The model under review builds one solid part; all positions refer to its coordinate system, in mm. A direction names the side the tool comes from. Round coordinates to 2 decimals unless told otherwise and drop trailing zeros. Write each loop counter-clockwise with the first axis right and the second up, starting at its lowest first coordinate (ties: lowest second). Pieces come first, ordered by that corner, then holes. Notation, with made-up numbers: (6, 74.5) - (30, 74.5) arc R20 cw to (30, 86.5) - close; hole circle Ø6 at (-32.75, 14.25). An arc over 180 degrees is marked (long way). Use one line per item in the form item = value.
from build123d import *

# Parameters (mm, degrees)
SKETCH1_W           = 20
SKETCH1_H           = 4.5
SKETCH2_R           = 1.5
CUT_EXTRUDE1_DEPTH  = 3
CHAMFER1_SIZE       = 0.3
SKETCH3_R           = 0.5
BOSS_EXTRUDE1_DEPTH = 5


with BuildPart() as part:
    # Sketch1 → Revolve1 (revolve)
    with BuildSketch(Plane(origin=(0, 0, 0), x_dir=(0, 0, -1), z_dir=(1, 0, 0)), mode=Mode.PRIVATE) as revolve1_sk:
        with Locations((0, 2.25)):
            Rectangle(SKETCH1_W, SKETCH1_H)
    revolve(revolve1_sk.sketch.rotate(Axis((0, 0, 10), (0, 0, -1)), 90), axis=Axis((0, 0, 10), (0, 0, -1)))

    # Sketch2 → Cut-Extrude1 (cut)
    with BuildSketch(Plane.XY.offset(10)):
        Circle(SKETCH2_R)
    extrude(amount=-CUT_EXTRUDE1_DEPTH, mode=Mode.SUBTRACT)

    # Chamfer1
    chamfer1_edges = [part.edges().sort_by_distance(p)[0] for p in [
        (-4.5, 0, -10),
        (-4.5, 0, 10),
    ]]
    chamfer(chamfer1_edges, length=CHAMFER1_SIZE)

    # Sketch3 → Boss-Extrude1 (add)
    with BuildSketch(Plane(origin=(0, 0, -10), x_dir=(-1, 0, 0), z_dir=(0, 0, -1))):
        with Locations(Location((-2, 0, 0), (0, 0, 180))):
            Circle(SKETCH3_R)
        with Locations(Location((2, 0, 0), (0, 0, 180))):
            Circle(SKETCH3_R)
    extrude(amount=BOSS_EXTRUDE1_DEPTH)


solid = part.part
(1) Add section D-D on z = -2.25. Write out the cut boundary in (x, y).
Geometry results:
outline = circle Ø9 at (0, 0)
(2) Add section A-A on x = 0. Write out the cut boundary in (y, z), then the cut area to 3 significant figures.
Geometry results:
outline = (-4.5, -9.7) - (-4.2, -10) - (4.2, -10) - (4.5, -9.7) - (4.5, 9.7) - (4.2, 10) - (1.5, 10) - (1.5, 7) - (-1.5, 7) - (-1.5, 10) - (-4.2, 10) - (-4.5, 9.7) - close
area = 171 mm2
(3) Machinability: for faces 4 (the flat face through (-2, 0, -15)), 5 (the cylindrical face through (1.5, 0, -12.5)), 6 (the flat face through (0, 0, 7)), which of the approach directions +Z, -Z, +X, -X, +Y, -Y give a long, thin tool a straight path to every point of the face, cutting with its end or side? Answer none if there is none.
Geometry results:
face_4 = -Z, +X, -X, +Y, -Y
face_5 = -Z
face_6 = +Z
(4) The part is to be moulded in two halves that separate along X. For faces 1 (the cylindrical face through (-3.32, -3.04, -0.14)), 2 (the flat face through (-2, 0, 10)), 3 (the cylindrical face through (-2.4, 0.3, -12.5)), say which applies: +X half, -X half, draft (parallel to the pull), parting line (faces both ways), or undercut.
Geometry results:
face_1 = parting line
face_2 = draft
face_3 = undercut
(5) Add section C-C on y = 0. Write out the cut boundary in (x, z), then the cut area to 3 significant figures.
Geometry results:
outline = (-4.5, -9.7) - (-4.2, -10) - (-2.5, -10) - (-2.5, -15) - (-1.5, -15) - (-1.5, -10) - (1.5, -10) - (1.5, -15) - (2.5, -15) - (2.5, -10) - (4.2, -10) - (4.5, -9.7) - (4.5, 9.7) - (4.2, 10) - (1.5, 10) - (1.5, 7) - (-1.5, 7) - (-1.5, 10) - (-4.2, 10) - (-4.5, 9.7) - close
area = 181 mm2
(6) Insertion check: P1, Ø2.5, axis at x = 0, y = 0, coming from the +Z side; P2, Ø5, axis at x = -2, y = -2, coming from the -Z side; P3, Ø4, axis at x = 3, y = 2.5, coming from the -Z side. Each pin has a flat end and moves straight along its axis. Give the tip position at first contact, or say it passes through.
Geometry results:
P1 = 7
P2 = -15
P3 = -10
(7) Add section B-B on z = 8.25. Write out the cut boundary in (x, y), then the cut area to 3 significant figures.
Geometry results:
outline = circle Ø9 at (0, 0); hole circle Ø3 at (0, 0)
area = 56.5 mm2
(8) To check wall thickness, follow L1, parallel to Y at x = 0, z = 8.8; L2, parallel to Z at x = 2, y = -1.25; L3, parallel to Z at x = -0.5, y = 1. State the ranges of each line that lie inside material, in increasing order.
Geometry results:
L1 = -4.5 to -1.5, 1.5 to 4.5
L2 = -10 to 10
L3 = -10 to 7
